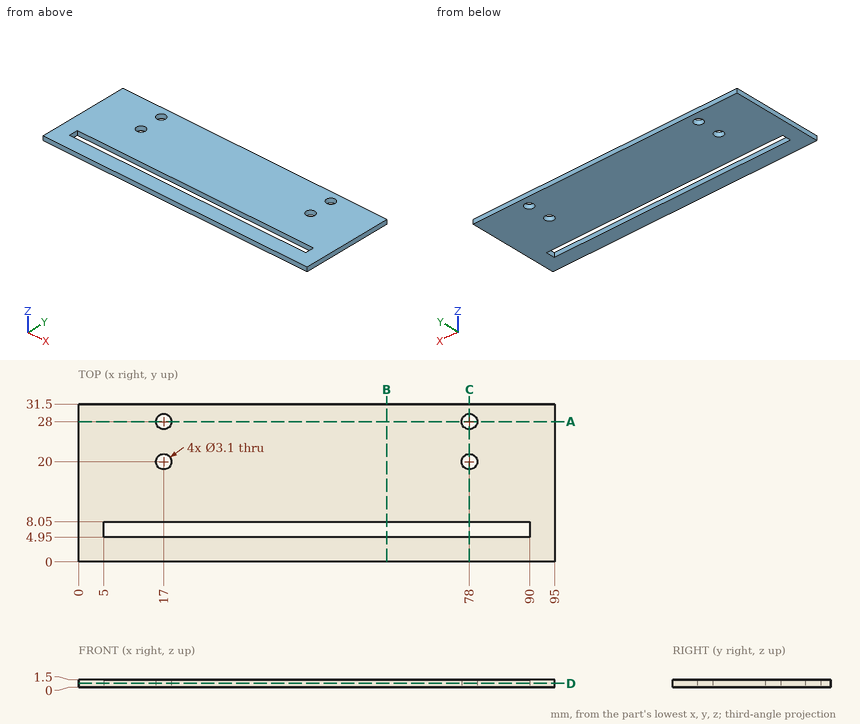
Can you work these out from the drawing? Everything is in mm from the part's minimum corner. Round coordinates to 2 decimals unless told otherwise and drop trailing zeros. Loops run counter-clockwise (first coordinate to the right, second up) from the corner with the lowest first, then second, coordinate; pieces in that order, holes last.
1. If we section it at B-B on x = 61.5: Write out the boundary of the cut face in (y, z), plus the area to 3 significant figures.
Answer list:
outline: (0, 0) - (4.95, 0) - (4.95, 1.5) - (0, 1.5) - close; (8.05, 0) - (31.5, 0) - (31.5, 1.5) - (8.05, 1.5) - close
area: 42.6 mm2
2. If we section it at A-A on y = 28: Write out the boundary of the cut face in (x, z), plus the area to 3 significant figures.
Answer list:
outline: (0, 0) - (15.45, 0) - (15.45, 1.5) - (0, 1.5) - close; (18.55, 0) - (76.45, 0) - (76.45, 1.5) - (18.55, 1.5) - close; (79.55, 0) - (95, 0) - (95, 1.5) - (79.55, 1.5) - close
area: 133 mm2
3. If we section it at C-C on x = 78: Write out the boundary of the cut face in (y, z).
Answer list:
outline: (0, 0) - (4.95, 0) - (4.95, 1.5) - (0, 1.5) - close; (8.05, 0) - (18.45, 0) - (18.45, 1.5) - (8.05, 1.5) - close; (21.55, 0) - (26.45, 0) - (26.45, 1.5) - (21.55, 1.5) - close; (29.55, 0) - (31.5, 0) - (31.5, 1.5) - (29.55, 1.5) - close
4. For P1, Ø3.5, axis at x = 17, y = 28, coming from the +Z side, with a flat end and sliding along its axis, tell me the tip position at first contact or that it passes through.
Answer list:
P1: stops at z = 1.5
5. If I drill on line 1 along X through (y, z) = (20, 0.7); line 2 along Y through (x, z) = (17, 0.5); line 3 along Y through (x, z) = (22, 1.3), over which ranges is the centre line in solid material (lowest first)?
Answer list:
line 1: x = 0 to 15.45, 18.55 to 76.45, 79.55 to 95
line 2: y = 0 to 4.95, 8.05 to 18.45, 21.55 to 26.45, 29.55 to 31.5
line 3: y = 0 to 4.95, 8.05 to 31.5
6. If we section it at D-D on z = 0.8: Write out the boundary of the cut face in (x, y), plus the area to 3 significant figures.
Answer list:
outline: (0, 0) - (95, 0) - (95, 31.5) - (0, 31.5) - close; hole (5, 4.95) - (90, 4.95) - (90, 8.05) - (5, 8.05) - close; hole circle Ø3.1 at (17, 20); hole circle Ø3.1 at (17, 28); hole circle Ø3.1 at (78, 20); hole circle Ø3.1 at (78, 28)
area: 2,700 mm2
